```python
from build123d import *

# Parameters (mm, degrees)
FILLET1_R = 0.15


with BuildPart() as part:
    # Sketch1 → Revolve1 (revolve)
    with BuildSketch(Plane.XY):
        Polygon((0, 19.9), (-0.735, 19.9), (-0.735, 15.9), (-0.99, 15.9), (-0.99, 0.94), (-0.75, 0.94), (-0.75, 0.5), (-0.99, 0.5), (-0.99, 0), (0, 0), align=None)
    revolve(axis=Axis((0, 19.9, 0), (0, -1, 0)))

    # Fillet1
    fillet1_edges = [part.edges().sort_by_distance(p)[0] for p in [
        (0.735, 15.9, 0),
        (0.735, 19.9, 0),
        (0.99, 0, 0),
    ]]
    fillet(fillet1_edges, radius=FILLET1_R)


solid = part.part
```
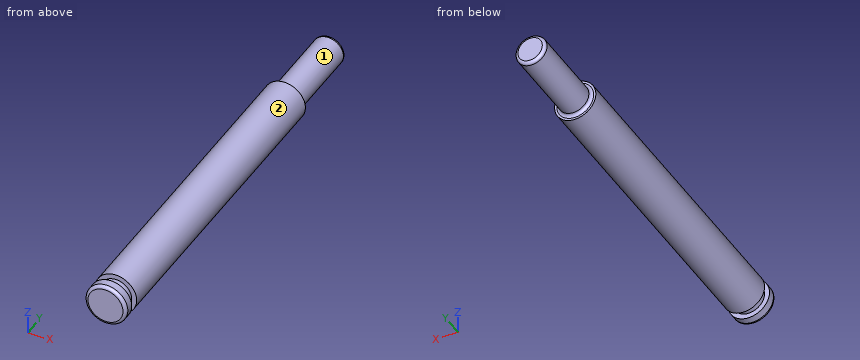
Design review of the part built by this model. Coordinates are the model's own, in mm. Face numbers are marked on the shaded views. A direction names the side the tool comes from. Coordinates: 2 decimals unless noted, no trailing zeros. Order: outer loops, then holes, each group sorted by start corner. A loop starts at its lowest first (then second) coordinate and runs counter-clockwise, first axis right, second up.
1) For the marked faces 1 and 2, list the 3-axis set-ups (+Z, -Z, +X, -X, +Y, -Y) from which the entire face can be reached by the end or side of a thin tool; tool diameter is ignored.
2) Take a section at C-C, the plane y = 14.5. Give the boundary of the cut face in (x, z).
3) Wall thickness on line 1 along X through (y, z) = (1, 0.65); line 2 along X through (y, z) = (6, 0.8); line 3 along Y through (x, z) = (0.8, -0.5): over which ranges is each line inside the solid? List them lowest first.
4) Take a section at A-A, the plane x = 0. Give the boundary of the cut face in (y, z) (3 decimals), and give its area (3 significant figures).
5) Take a section at D-D, the plane y = 17.25. Give the boundary of the cut face in (x, z) (3 decimals), and give its area (3 significant figures).
6) Take a section at B-B, the plane z = 0. Give the boundary of the cut face in (x, y) (3 decimals).
Returned:
1. face 1: +Y
1. face 2: +Y, -Y
2. outline: circle Ø1.98 at (0, 0)
3. line 1: x = -0.75 to 0.75
3. line 2: x = -0.58 to 0.58
3. line 3: y = 0.04 to 0.5, 0.94 to 15.9
4. outline: (0, -0.84) arc R0.15 ccw to (0.15, -0.99) - (0.5, -0.99) - (0.5, -0.75) - (0.94, -0.75) - (0.94, -0.99) - (15.9, -0.99) - (15.9, -0.885) arc R0.15 cw to (16.05, -0.735) - (19.75, -0.735) arc R0.15 ccw to (19.9, -0.585) - (19.9, 0.585) arc R0.15 ccw to (19.75, 0.735) - (16.05, 0.735) arc R0.15 cw to (15.9, 0.885) - (15.9, 0.99) - (0.94, 0.99) - (0.94, 0.75) - (0.5, 0.75) - (0.5, 0.99) - (0.15, 0.99) arc R0.15 ccw to (0, 0.84) - close
4. area: 37.1 mm2
5. outline: circle Ø1.47 at (0, 0)
5. area: 1.70 mm2
6. outline: (-0.99, 0.15) arc R0.15 ccw to (-0.84, 0) - (0.84, 0) arc R0.15 ccw to (0.99, 0.15) - (0.99, 0.5) - (0.75, 0.5) - (0.75, 0.94) - (0.99, 0.94) - (0.99, 15.9) - (0.885, 15.9) arc R0.15 cw to (0.735, 16.05) - (0.735, 19.75) arc R0.15 ccw to (0.585, 19.9) - (-0.585, 19.9) arc R0.15 ccw to (-0.735, 19.75) - (-0.735, 16.05) arc R0.15 cw to (-0.885, 15.9) - (-0.99, 15.9) - (-0.99, 0.94) - (-0.75, 0.94) - (-0.75, 0.5) - (-0.99, 0.5) - close
